The model under review builds one solid part; all positions refer to its coordinate system, in mm. Coordinates: 2 decimals unless noted, no trailing zeros. Write each loop counter-clockwise with the first axis right and the second up, starting at its lowest first coordinate (ties: lowest second). Pieces come first, ordered by that corner, then holes. Notation, with made-up numbers: (69.25, 49) - (100.25, 49) arc R20 cw to (100.25, 74) - close; hole circle Ø9 at (-34, -8). An arc over 180 degrees is marked (long way). Return JSON: item names as keys, results as strings. Group by question number.
(1) We need section A-A on z = -25.4. State the section outline as (x, y) points.
(2) To check wall thickness, follow L1, parallel to Z at x = 0.8, y = 0; L2, parallel to Z at x = 0.1, y = 0.75; L3, parallel to Y at x = 1.4, z = 1. State the ranges of each line that lie inside material, in increasing order. Write a range as from..to.
(3) We need section D-D on y = 3.5. State the section outline as (x, z) points.
(4) We need section C-C on x = 0.55. State the section outline as (y, z) points (1 decimal), then the cut area to 3 significant figures.
(5) Draft analysis for pull direction Z (two halves, no side actions). For faces 1 (the face through (1.588, 0, -19)), 2 (the face through (0.783, 2.003, -0.631)), 3 (the face through (0.78, 0.1, -42.86)), state which applies: released by +Z, released by -Z, zero draft, split by the parting line, or undercut.
(6) We need section B-B on y = 0. State the section outline as (x, z) points.
(7) For pin 1 Ø1 at (y, z) = (2, -16.5) entering from -X; pin 2 Ø3.5 at (y, z) = (0, -38.1) entering from +X, all flat-tipped, find the tip position at first contact; note any pin that passes through.
Autodesk Inventor part; units mm, degrees
ref_plane "YZ Plane" through (0, 0, 0) normal (1, 0, 0) x (0, 1, 0)
ref_plane "XZ Plane" through (0, 0, 0) normal (0, 1, 0) x (-1, 0, 0)
ref_plane "XY Plane" through (0, 0, 0) normal (0, 0, 1) x (1, 0, 0)
sketch "Sketch1" plane through (0, 0, 0) normal (1, 0, 0) x (0, 1, 0)
  circle A0 centre (0, 0) radius 2.1
  circle A1 centre (0, -25.4) radius 2.0828
  circle A2 centre (0, -38.1) radius 2.1
  arc A3 (4.7625, 0) -> (-4.7625, 0) centre (0, 0) ccw
  arc A4 (-4.7625, -38.1) -> (4.7625, -38.1) centre (0, -38.1) ccw
  line L0 (4.7625, 0) -> (4.7625, -38.1)
  line L1 (-4.7625, 0) -> (-4.7625, -38.1)
  dimension "d0" = 4.2
  dimension "d4" = 4.1656
  dimension "d5" = 4.2
extrude "Extrusion1" add sketch "Sketch1" along normal blind 1.5875
properties part number "Gearbox Gusset" material "Acetal Resin, White"
Ans:
{
 "1": {"outline": "(0, -4.76) - (1.59, -4.76) - (1.59, -2.08) - (0, -2.08) - close; (0, 2.08) - (1.59, 2.08) - (1.59, 4.76) - (0, 4.76) - close"},
 "2": {"L1": "-42.86..-40.2, -36..-27.48, -23.32..-2.1, 2.1..4.76", "L2": "-42.8..-40.06, -36.14..-27.34, -23.46..-1.96, 1.96..4.7", "L3": "-4.66..-1.85, 1.85..4.66"},
 "3": {"outline": "(0, -41.33) - (1.59, -41.33) - (1.59, 3.23) - (0, 3.23) - close"},
 "4": {"outline": "(-4.8, -38.1) arc R4.8 ccw to (4.8, -38.1) - (4.8, 0) arc R4.8 ccw to (-4.8, 0) - close; hole circle Ø4.2 at (0, -38.1); hole circle Ø4.2 at (0, -25.4); hole circle Ø4.2 at (0, 0)", "area": "393 mm²"},
 "5": {"face 1": "zero draft", "face 2": "undercut", "face 3": "released by -Z"},
 "6": {"outline": "(0, -42.86) - (1.59, -42.86) - (1.59, -40.2) - (0, -40.2) - close; (0, -36) - (1.59, -36) - (1.59, -27.48) - (0, -27.48) - close; (0, -23.32) - (1.59, -23.32) - (1.59, -2.1) - (0, -2.1) - close; (0, 2.1) - (1.59, 2.1) - (1.59, 4.76) - (0, 4.76) - close"},
 "7": {"pin 1": "x = 0", "pin 2": "through"}
}
